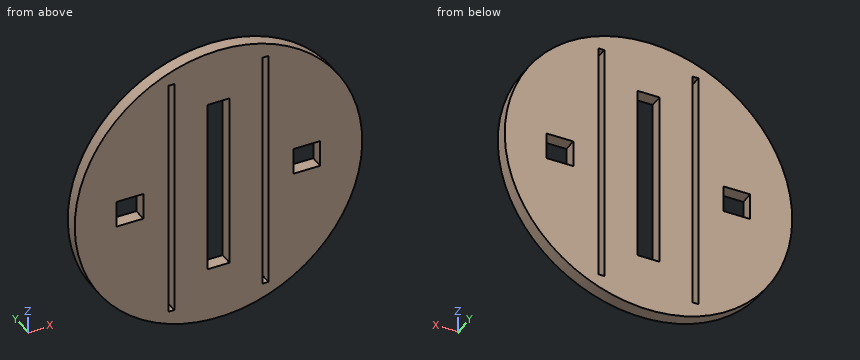
```python
from build123d import *

# Parameters (mm, degrees)
SKETCH1_R               = 32.5
BOSS_EXTRUDE1_DEPTH     = 3
CUT_EXTRUDE1_DEPTH      = 27.5
CUT_EXTRUDE1_DEPTH_BACK = 27.5
SKETCH2_W               = 1.3
SKETCH2_H               = 6.728638504
SKETCH3_W               = 6
SKETCH3_H               = 6
CUT_EXTRUDE2_DEPTH      = 10
SKETCH4_W               = 5
SKETCH4_H               = 40
CUT_EXTRUDE3_DEPTH      = 10


with BuildPart() as part:
    # Sketch1 → Boss-Extrude1 (new body)
    with BuildSketch(Plane(origin=(0, 0, 0), x_dir=(1, 0, 0), z_dir=(0, 1, 0))):
        with Locations(Location((0, 0, 0), (0, 0, 270))):
            Circle(SKETCH1_R)
    extrude(amount=BOSS_EXTRUDE1_DEPTH)

    # Sketch2 → Cut-Extrude1 (cut, two sides: drawn at the far end of the back side and taken through both)
    with BuildSketch(Plane.XY.offset(-CUT_EXTRUDE1_DEPTH_BACK)):
        with Locations((-10.65, 0)):
            Rectangle(SKETCH2_W, SKETCH2_H)
        with Locations((10.65, 0)):
            Rectangle(SKETCH2_W, SKETCH2_H)
    extrude(amount=CUT_EXTRUDE1_DEPTH + CUT_EXTRUDE1_DEPTH_BACK, mode=Mode.SUBTRACT)

    # Sketch3 → Cut-Extrude2 (cut)
    with BuildSketch(Plane(origin=(0, 0, 0), x_dir=(1, 0, 0), z_dir=(0, 1, 0))):
        with Locations((-20, 0)):
            Rectangle(SKETCH3_W, SKETCH3_H)
        with Locations((20, 0)):
            Rectangle(SKETCH3_W, SKETCH3_H)
    extrude(amount=CUT_EXTRUDE2_DEPTH, mode=Mode.SUBTRACT)

    # Sketch4 → Cut-Extrude3 (cut)
    with BuildSketch(Plane.XZ):
        Rectangle(SKETCH4_W, SKETCH4_H)
    extrude(amount=-CUT_EXTRUDE3_DEPTH, mode=Mode.SUBTRACT)


solid = part.part
```
Geometry check sheet. Reference: the model listing, model coordinates, mm. Round coordinates to 2 decimals unless told otherwise and drop trailing zeros. Write each loop counter-clockwise with the first axis right and the second up, starting at its lowest first coordinate (ties: lowest second). Pieces come first, ordered by that corner, then holes. Notation, with made-up numbers: (59.25, 43.25) -> (77.25, 43.25) arc R29 ccw to (77.25, 69.25) -> close; hole circle Ø7 at (13.5, 4). An arc over 180 degrees is marked (long way). Put each result on its own line as item: value.
1) Cross-section at C-C, the plane x = 0. Enter the section's corners in (y, z), plus the area to 3 significant figures.
Recorded:
outline: (0, -32.5) -> (3, -32.5) -> (3, -20) -> (0, -20) -> close; (0, 20) -> (3, 20) -> (3, 32.5) -> (0, 32.5) -> close
area: 75.0 mm2
2) Cross-section at D-D, the plane z = -15. Enter the section's corners in (x, y).
Recorded:
outline: (-28.83, 0) -> (-11.3, 0) -> (-11.3, 3) -> (-28.83, 3) -> close; (-10, 0) -> (-2.5, 0) -> (-2.5, 3) -> (-10, 3) -> close; (2.5, 0) -> (10, 0) -> (10, 3) -> (2.5, 3) -> close; (11.3, 0) -> (28.83, 0) -> (28.83, 3) -> (11.3, 3) -> close
3) Cross-section at B-B, the plane z = 0. Enter the section's corners in (x, y), plus the area to 3 significant figures.
Recorded:
outline: (-32.5, 0) -> (-23, 0) -> (-23, 3) -> (-32.5, 3) -> close; (-17, 0) -> (-11.3, 0) -> (-11.3, 3) -> (-17, 3) -> close; (-10, 0) -> (-2.5, 0) -> (-2.5, 3) -> (-10, 3) -> close; (2.5, 0) -> (10, 0) -> (10, 3) -> (2.5, 3) -> close; (11.3, 0) -> (17, 0) -> (17, 3) -> (11.3, 3) -> close; (23, 0) -> (32.5, 0) -> (32.5, 3) -> (23, 3) -> close
area: 136 mm2
4) Thickness scan on probe 1 along X at (y, z) = (1.9, 7.5); probe 2 along X at (y, z) = (2.25, -9); probe 3 along X at (y, z) = (2.2, 0). Record the ranges inside material, lowest first. Write a range as from..to.
Recorded:
probe 1: x = -31.62..-11.3, -10..-2.5, 2.5..10, 11.3..31.62
probe 2: x = -31.23..-11.3, -10..-2.5, 2.5..10, 11.3..31.23
probe 3: x = -32.5..-23, -17..-11.3, -10..-2.5, 2.5..10, 11.3..17, 23..32.5
5) Depth check by flat-ended pin: P1, Ø0.9, axis at y = 2, z = 0, coming from the -X side; P2, Ø1, axis at x = 10.5, y = 1, coming from the +Z side; P3, Ø1.5, axis at x = 2.5, y = 2.5, coming from the -Z side. Enter the tip coordinate at first touch or a pass-through.
Recorded:
P1: stops at x = -32.5
P2: stops at z = 30.92
P3: stops at z = -32.45
6) Cross-section at A-A, the plane y = 0.7. Enter the section's corners in (x, z), plus the area to 3 significant figures.
Recorded:
outline: circle Ø65 at (0, 0); hole (-23, -3) -> (-17, -3) -> (-17, 3) -> (-23, 3) -> close; hole (-11.3, -27.5) -> (-10, -27.5) -> (-10, 27.5) -> (-11.3, 27.5) -> close; hole (-2.5, -20) -> (2.5, -20) -> (2.5, 20) -> (-2.5, 20) -> close; hole (10, -27.5) -> (11.3, -27.5) -> (11.3, 27.5) -> (10, 27.5) -> close; hole (17, -3) -> (23, -3) -> (23, 3) -> (17, 3) -> close
area: 2,900 mm2
